Study the drawing (mm; zero at the part's minimum x, y, z) and answer. A direction names the side the tool comes from. Give positions to 0.01 mm unless a question says otherwise; leave off trailing zeros. Loops run counter-clockwise (first coordinate to the right, second up) from the corner with the lowest first, then second, coordinate; pieces in that order, holes last. Notation, with made-up numbers: (84.25, -29) - (126.25, -29) arc R32 ccw to (126.25, 8) - close; hole circle Ø7 at (11.5, -30.5). An arc over 180 degrees is marked (long way). Answer in a Markdown table with one row per item. Add a question column.
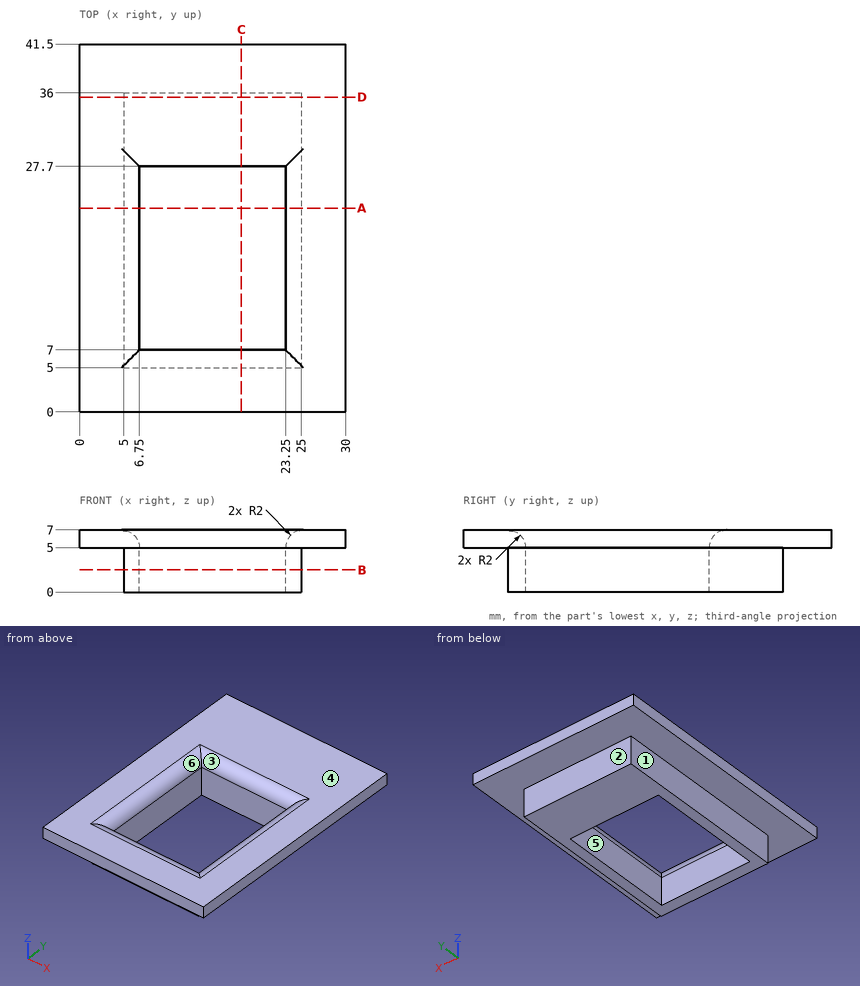
(1) Given pin 1 Ø2.5 at (x, z) = (20, 3) entering from -Y; pin 2 Ø2.5 at (y, z) = (13.5, 1.5) entering from +X; pin 3 Ø1.5 at (y, z) = (16, 2) entering from -X; pin 4 Ø4 at (y, z) = (26, 3.5) entering from -X, each flat-ended and moving along its own axis, determine where each tip first touches the part or whether it passes through.
(2) A cutting plane is placed at A-A on y = 23. Determine the outline of the cut face in (x, z).
(3) A cutting plane is placed at C-C on x = 18.25. Determine the outline of the cut face in (y, z).
(4) A tool of negligible diameter and unlimited length cuts with its end or side. For the marked faces 4, 5 and 6, from which of +Z, -Z, +X, -X, +Y, -Y can it reach the whole face along a straight path? Write none if from no direction.
(5) A cutting plane is placed at D-D on y = 35.5. Determine the outline of the cut face in (x, z).
(6) A cutting plane is placed at B-B on z = 2.5. Determine the outline of the cut face in (x, y), plus the area to 3 significant figures.
(7) Find the intervals of material crossed by line 1 along Y through (x, z) = (16.25, 3.75); line 2 along X through (y, z) = (17, 2.5); line 3 along X through (y, z) = (34.5, 3), in increasing order. Write a range as [from, to].
(8) The mould has two halves that part along X. Classify the marked faces 1, 2 and 3: pulls with the +X half, pulls with the -X half, needs draft (parallel to the pull), parting line crosses it, or undercut.
Evaluation:
| question | item | result |
|---|---|---|
| 1 | pin 1 | stops at y = 5 |
| 1 | pin 2 | stops at x = 25 |
| 1 | pin 3 | stops at x = 5 |
| 1 | pin 4 | stops at x = 0 |
| 2 | outline | (0, 5) - (5, 5) - (5, 0) - (6.75, 0) - (6.75, 5) arc R2 ccw to (4.75, 7) - (0, 7) - close; (23.25, 0) - (25, 0) - (25, 5) - (30, 5) - (30, 7) - (25.25, 7) arc R2 ccw to (23.25, 5) - close |
| 3 | outline | (0, 5) - (5, 5) - (5, 0) - (7, 0) - (7, 5) arc R2 ccw to (5, 7) - (0, 7) - close; (27.7, 0) - (36, 0) - (36, 5) - (41.5, 5) - (41.5, 7) - (29.7, 7) arc R2 ccw to (27.7, 5) - close |
| 4 | face 4 | +Z, +X, -X, +Y, -Y |
| 4 | face 5 | +Z, -Z |
| 4 | face 6 | +Z |
| 5 | outline | (0, 5) - (5, 5) - (5, 0) - (25, 0) - (25, 5) - (30, 5) - (30, 7) - (0, 7) - close |
| 6 | outline | (5, 5) - (25, 5) - (25, 36) - (5, 36) - close; hole (6.75, 7) - (23.25, 7) - (23.25, 27.7) - (6.75, 27.7) - close |
| 6 | area | 278 mm² |
| 7 | line 1 | y = [5, 7], [27.7, 36] |
| 7 | line 2 | x = [5, 6.75], [23.25, 25] |
| 7 | line 3 | x = [5, 25] |
| 8 | face 1 | pulls with the -X half |
| 8 | face 2 | needs draft |
| 8 | face 3 | undercut |
